```python
from build123d import *

# Parameters (mm, degrees)
F1_DEPTH = 18
F4_R     = 11
F5_DEPTH = 18.001
F6_SIZE  = 1


# Not quite as in the source:
# - a feature names something its author has since deleted; it is built from what else it names


with BuildPart() as f1:
    # F0 (on Top) → F1 (new body)
    with BuildSketch(Plane.XY):
        Polygon((18.4752086141, 0), (9.237604307, 16), (-9.237604307, 16), (-18.4752086141, 0), (-9.237604307, -16), (9.237604307, -16), align=None)
    extrude(amount=F1_DEPTH)

    # F2 (on Right) → F3 (revolve, cut)
    with BuildSketch(Plane.YZ):
        Polygon((-29.0477817086, 10.4668597182), (-16, 18), (-29.0477817086, 18), align=None)
        Polygon((-16, 0), (-29.0477817086, 7.5331402818), (-29.0477817086, 0), align=None)
    revolve(axis=Axis((0, 0, 10.077371262), (0, 0, 1)), mode=Mode.SUBTRACT)

    # F4 (on face) → F5 (cut, through all)
    with BuildSketch(Plane(origin=(0, 0, 0), x_dir=(1, 0, 0), z_dir=(0, 0, -1))):
        Circle(F4_R)
    extrude(amount=-F5_DEPTH, mode=Mode.SUBTRACT)

    # F6
    f6_edges = [f1.edges().sort_by_distance(p)[0] for p in [
        (-11, 0, 0),
        (-11, 0, 18),
    ]]
    chamfer(f6_edges, length=F6_SIZE)


solid = f1.part
```
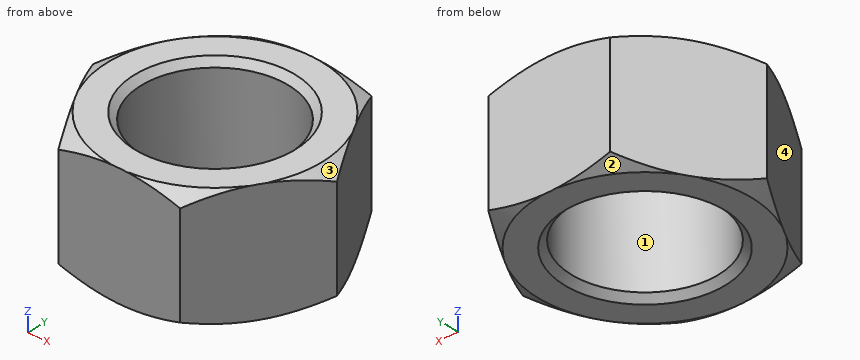
Design review of the part built by this model. Coordinates are the model's own, in mm. Face numbers are marked on the shaded views. Coordinates: 2 decimals unless noted, no trailing zeros. Order: outer loops, then holes, each group sorted by start corner. A loop starts at its lowest first (then second) coordinate and runs counter-clockwise, first axis right, second up. Notation, with made-up numbers: (87.5, 61) - (132.5, 61) arc R12 ccw to (132.5, 67) - close; hole circle Ø4 at (9, 17.25). An arc over 180 degrees is marked (long way). One line per question, with ' | ' between items.
Q1. The part is to be moulded in two halves that separate along Y. For the marked faces 1, 2, 3 and 4, say which applies: +Y half, -Y half, draft (parallel to the pull), parting line (faces both ways), or undercut.
Answer key:
face 1: undercut | face 2: +Y half | face 3: parting line | face 4: -Y half
Q2. Consider section A-A, the plane z = 8.5. Give the boundary of the cut face in (x, y).
Answer key:
outline: (-18.48, 0) - (-9.24, -16) - (9.24, -16) - (18.48, 0) - (9.24, 16) - (-9.24, 16) - close; hole circle Ø22 at (0, 0)
Q3. To check wall thickness, follow line 1 along X through (y, z) = (0, 7.25); line 2 along X through (y, z) = (3, 8.5); line 3 along Y through (x, z) = (7, 7). State the ranges of each line that lie inside material, in increasing order.
Answer key:
line 1: x = -18.48 to -11, 11 to 18.48 | line 2: x = -16.74 to -10.58, 10.58 to 16.74 | line 3: y = -16 to -8.49, 8.49 to 16
Q4. Clearance check with flat-ended pins moving along their axes: pin 1 Ø5 at (x, z) = (10, 13.5) entering from -Y; pin 2 Ø2 at (y, z) = (-3.5, 12.5) entering from -X; pin 3 Ø3 at (y, z) = (11.5, 7.5) entering from +X; pin 4 Ø6 at (y, z) = (3.5, 5.5) entering from +X. State where each tip first meets the part, or that it passes through.
Answer key:
pin 1: stops at y = -16 | pin 2: stops at x = -17.03 | pin 3: stops at x = 12.7 | pin 4: stops at x = 18.19
